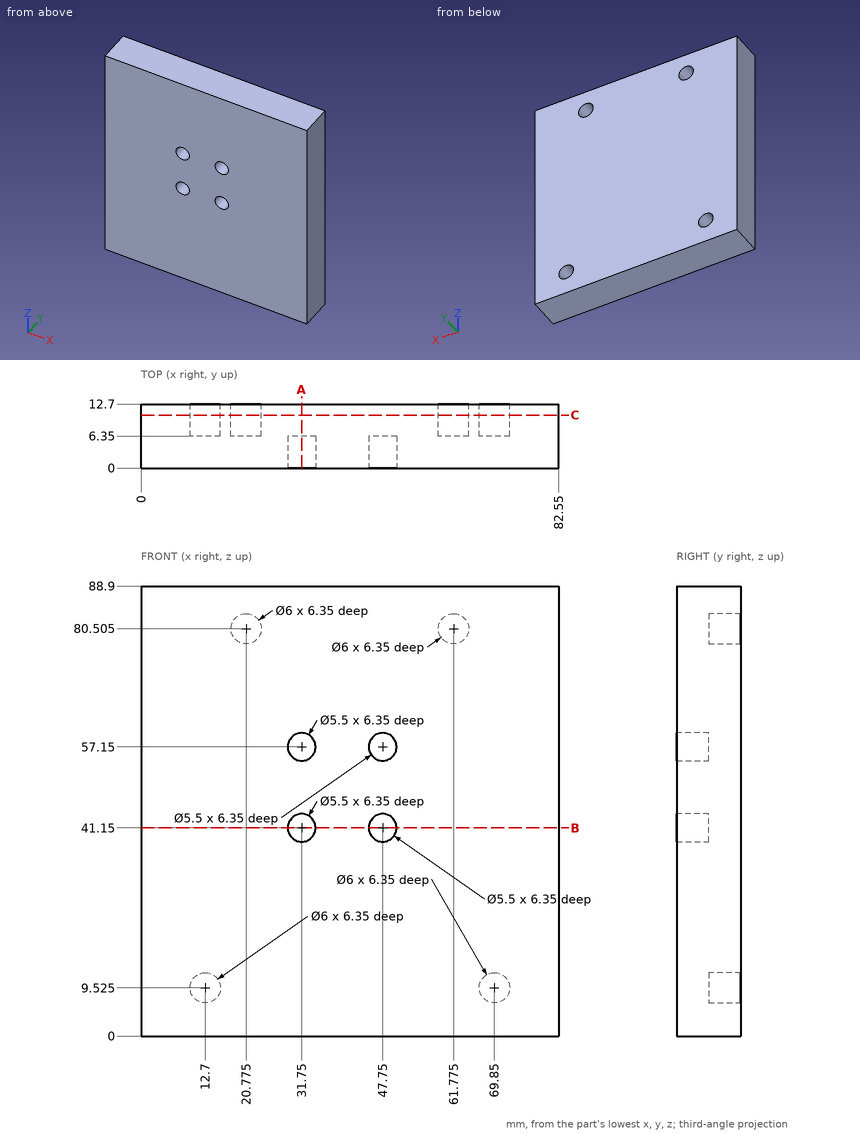
For this review, use the dimensioned drawing (mm, ordinates from the lowest corner) and the shaded views. Coordinates: 2 decimals unless noted, no trailing zeros. Write each loop counter-clockwise with the first axis right and the second up, starting at its lowest first coordinate (ties: lowest second). Pieces come first, ordered by that corner, then holes. Notation, with made-up numbers: (39, 37) -> (74, 37) arc R23 ccw to (74, 59) -> close; hole circle Ø9 at (-1.5, 66). An arc over 180 degrees is marked (long way). Put each result on its own line as item: value.
Q1. Take a section at C-C, the plane y = 10.5. Count the separate pieces of the cut face and the enclosed holes in it, then the cut area to 3 significant figures.
From the geometry:
separate pieces: 1
enclosed holes: 4
area: 7,230 mm2
Q2. Take a section at B-B, the plane z = 41.15. State the section outline as (x, y) points.
From the geometry:
outline: (0, 0) -> (29, 0) -> (29, 6.35) -> (34.5, 6.35) -> (34.5, 0) -> (45, 0) -> (45, 6.35) -> (50.5, 6.35) -> (50.5, 0) -> (82.55, 0) -> (82.55, 12.7) -> (0, 12.7) -> close
Q3. Clearance check with flat-ended pins moving along their axes: pin 1 Ø1.8 at (x, z) = (21.5, 81.5) entering from +Y; pin 2 Ø3 at (x, z) = (31.5, 57) entering from -Y. State where each tip first meets the part, or that it passes through.
From the geometry:
pin 1: stops at y = 6.35
pin 2: stops at y = 6.35
Q4. Wall thickness on L1, parallel to X at y = 1.5, z = 57.15; L2, parallel to X at y = 5.5, z = 39.5: over which ranges is each line inside the solid? List them lowest first.
From the geometry:
L1: x = 0 to 29, 34.5 to 45, 50.5 to 82.55
L2: x = 0 to 29.55, 33.95 to 45.55, 49.95 to 82.55
Q5. Take a section at A-A, the plane x = 31.75. State the section outline as (y, z) points.
From the geometry:
outline: (0, 0) -> (12.7, 0) -> (12.7, 88.9) -> (0, 88.9) -> (0, 59.9) -> (6.35, 59.9) -> (6.35, 54.4) -> (0, 54.4) -> (0, 43.9) -> (6.35, 43.9) -> (6.35, 38.4) -> (0, 38.4) -> close
